Could you check a few things on this model? Use its own coordinates, in mm. Face numbers are marked on the shaded views. Coordinates: 2 decimals unless noted, no trailing zeros. Loops run counter-clockwise (first coordinate to the right, second up) from the corner with the lowest first, then second, coordinate; pieces in that order, holes last. Notation, with made-up numbers: (52.25, 30) -> (101.25, 30) arc R14 cw to (101.25, 44) -> close; hole circle Ø6 at (35.25, 35). An arc over 180 degrees is marked (long way). One line per question, with ' | ' between items.
from build123d import *

# Parameters (mm, degrees)
SKETCH1_R               = 2.067
BASENUT_DEPTH           = 4.7
ENDCHAMFER_SIZE         = 0.433
ENDCHAMFER_SIZE2        = 0.249992667
ENDCHAMFER_PART_2_SIZE  = 0.433
ENDCHAMFER_PART_2_SIZE2 = 0.249992667


with BuildPart() as part:
    # Sketch1 → BaseNut (new body)
    with BuildSketch(Plane.XY):
        Polygon((4.618802154, 0), (2.309401077, 4), (-2.309401077, 4), (-4.618802154, 0), (-2.309401077, -4), (2.309401077, -4), align=None)
        Circle(SKETCH1_R, mode=Mode.SUBTRACT)
    extrude(amount=-BASENUT_DEPTH)

    # Sketch2 → Double-Chamfer (revolve, cut)
    with BuildSketch(Plane(origin=(0, 0, 0), x_dir=(1, 0, 0), z_dir=(0, 1, 0))):
        Polygon((-4.618802154, 4.7), (-3.625, 4.7), (-4.618802154, 4.126228059), align=None)
        Polygon((-4.618802154, 0.573771941), (-4.618802154, 0), (-3.625, 0), align=None)
    revolve(axis=Axis((0, 0, -3.375940562), (0, 0, 1)), mode=Mode.SUBTRACT)

    # EndChamfer
    endchamfer_edges = [part.edges().sort_by_distance(p)[0] for p in [
        (-2.067, 0, -4.7),
    ]]
    endchamfer_side = [part.faces().sort_by_distance(p)[0] for p in [
        (-2.067, 0, -2.35),
    ]]
    chamfer(endchamfer_edges, length=ENDCHAMFER_SIZE, length2=ENDCHAMFER_SIZE2, reference=endchamfer_side[0])

    # EndChamfer part 2
    endchamfer_part_2_edges = [part.edges().sort_by_distance(p)[0] for p in [
        (-2.067, 0, 0),
    ]]
    endchamfer_part_2_side = [part.faces().sort_by_distance(p)[0] for p in [
        (3.522469517, 0, 0),
    ]]
    chamfer(endchamfer_part_2_edges, length=ENDCHAMFER_PART_2_SIZE, length2=ENDCHAMFER_PART_2_SIZE2, reference=endchamfer_part_2_side[0])


solid = part.part
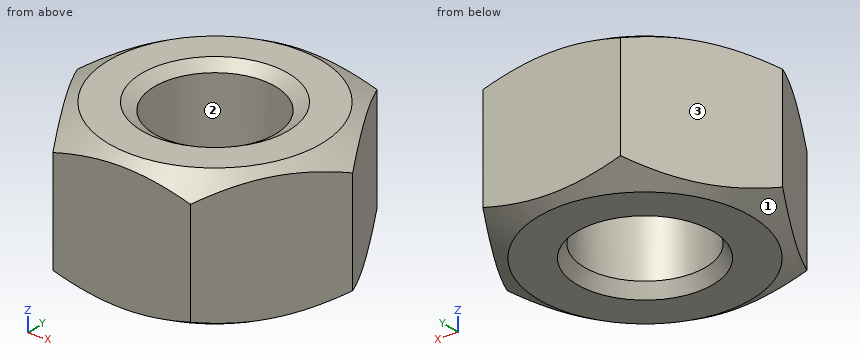
1) If we section it at B-B on z = -0.7: Please give me the cut outline in (x, y), and give its area (3 significant figures).
Data:
outline: (-4.62, 0) -> (-2.31, -4) -> (2.31, -4) -> (4.62, 0) -> (2.31, 4) -> (-2.31, 4) -> close; hole circle Ø4.13 at (0, 0) | area: 42.0 mm²
2) We'd pull the mould along Y, two halves only. Please class the marked faces 1, 2 and 3: pulls with the +Y half, pulls with the -Y half, needs draft (parallel to the pull), parting line crosses it, or undercut.
Data:
face 1: parting line crosses it | face 2: undercut | face 3: pulls with the +Y half
3) I need wall thicknesses on line 1 along Y through (x, z) = (0, -1.6); line 2 along X through (y, z) = (-0.25, -2.4); line 3 along Y through (x, z) = (1.25, -2.35). Which ranges of each line are inside material? Lowest first, please. Write a range as from..to.
Data:
line 1: -4..-2.07, 2.07..4 | line 2: -4.47..-2.05, 2.05..4.47 | line 3: -4..-1.65, 1.65..4
4) I'm going to push flat-ended pins straight in: pin 1 Ø1 at (x, z) = (-3, -2) entering from -Y; pin 2 Ø1.5 at (y, z) = (1.5, -3) entering from +X. Where does each tip first touch, or does it pass through?
Data:
pin 1: y = -3.67 | pin 2: x = 4.19
